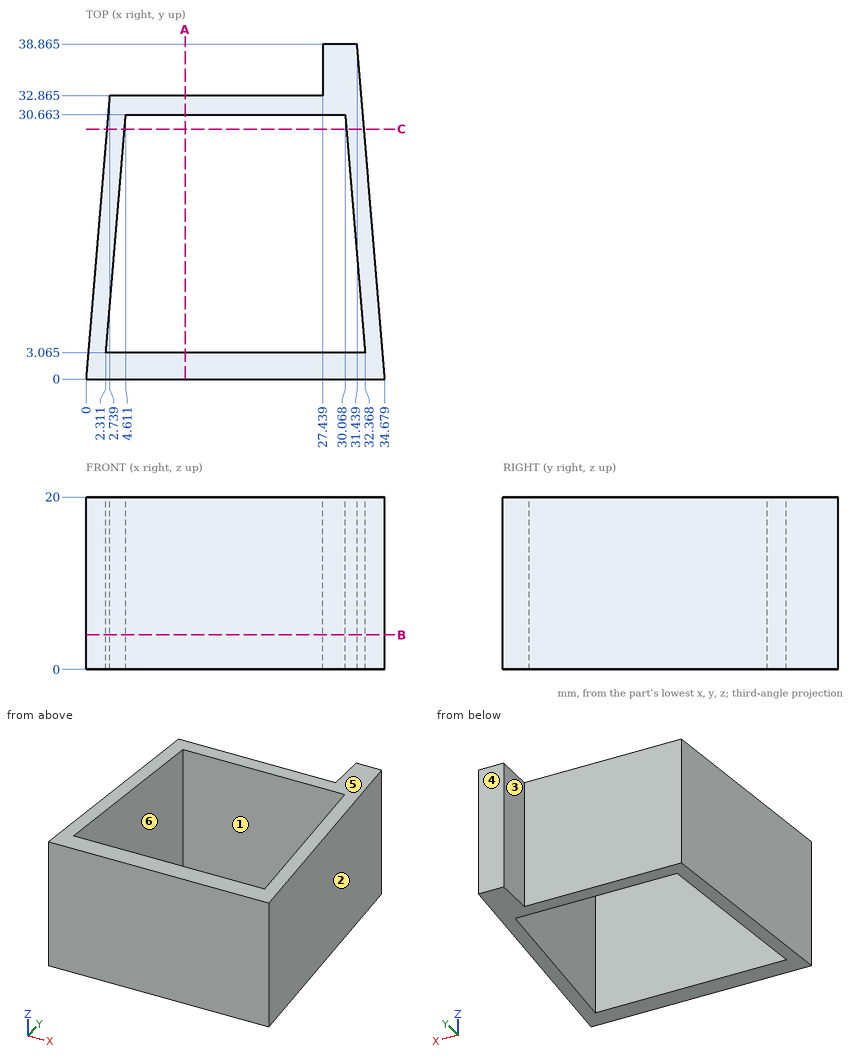
Drawing for the job (mm, zero at the part's lowest x, y, z). A direction names the side the tool comes from. Coordinates: 2 decimals unless noted, no trailing zeros. Order: outer loops, then holes, each group sorted by start corner. A loop starts at its lowest first (then second) coordinate and runs counter-clockwise, first axis right, second up. Notation, with made-up numbers: (20.25, 66) -> (30.25, 66) arc R28 cw to (30.25, 92) -> close; hole circle Ø10 at (59, 85). An arc over 180 degrees is marked (long way). Answer in a Markdown table with one row per item.
1) Which spindle directions (+Z, -Z, +X, -X, +Y, -Y) get a long thin tool onto all of the face, cutting with end or side? Do the marked faces 1, 2 and 3. Say none if no direction does.
Check values:
| item | result |
|---|---|
| face 1 | +Z, -Z |
| face 2 | +Z, -Z, +X, +Y |
| face 3 | +Z, -Z, -X, +Y |
2) Band-saw the part on A-A (x = 11.5). List the corners of the cut face in (y, z) (1 decimal), and give its area (3 significant figures).
Check values:
| item | result |
|---|---|
| outline | (0, 0) -> (3.1, 0) -> (3.1, 20) -> (0, 20) -> close; (30.7, 0) -> (32.9, 0) -> (32.9, 20) -> (30.7, 20) -> close |
| area | 105 mm2 |
3) Band-saw the part on B-B (z = 4). List the corners of the cut face in (x, y) (1 decimal), and give its area (3 significant figures).
Check values:
| item | result |
|---|---|
| outline | (0, 0) -> (34.7, 0) -> (31.4, 38.9) -> (27.4, 38.9) -> (27.4, 32.9) -> (2.7, 32.9) -> close; hole (2.3, 3.1) -> (32.4, 3.1) -> (30.1, 30.7) -> (4.6, 30.7) -> close |
| area | 309 mm2 |
4) Band-saw the part on C-C (y = 29). List the corners of the cut face in (x, z).
Check values:
| item | result |
|---|---|
| outline | (2.42, 0) -> (4.47, 0) -> (4.47, 20) -> (2.42, 20) -> close; (30.21, 0) -> (32.26, 0) -> (32.26, 20) -> (30.21, 20) -> close |
5) Flat gauge pins, fed straight in: P1, Ø6, axis at x = 24.5, z = 10.5, coming from the +Y side (1 decimal); P2, Ø10, axis at y = 29.5, z = 6.5, coming from the +X side; P3, Ø12, axis at y = 20.5, z = 13, coming from the +X side; P4, Ø3, axis at x = 24, z = 13, coming from the +Y side (1 decimal). Where does each tip first touch, or does it go through?
Check values:
| item | result |
|---|---|
| P1 | y = 38.9 |
| P2 | x = 32.64 |
| P3 | x = 33.47 |
| P4 | y = 32.9 |
6) Drill centre lines: line 1 (Y direction, x = 26.5, z = 11.25) (1 decimal); line 2 (Y direction, x = 28, z = 9) (1 decimal); line 3 (X direction, y = 17.5, z = 10.75) (1 decimal). Where is each one in solid material? Low to high.
Check values:
| item | result |
|---|---|
| line 1 | 0 to 3.1, 30.7 to 32.9 |
| line 2 | 0 to 3.1, 30.7 to 38.9 |
| line 3 | 1.5 to 3.5, 31.2 to 33.2 |
7) Mould opens along Y. For the marked faces 4, 5 and 6 say: pulls with the +Y half, pulls with the -Y half, needs draft (parallel to the pull), parting line crosses it, or undercut.
Check values:
| item | result |
|---|---|
| face 4 | pulls with the +Y half |
| face 5 | needs draft |
| face 6 | undercut |
